Source: CAD feature listing. Evaluate the final solid. Frame: model axes, mm. Round coordinates to 2 decimals unless told otherwise and drop trailing zeros. Loops run counter-clockwise (first coordinate to the right, second up) from the corner with the lowest first, then second, coordinate; pieces in that order, holes last. Notation, with made-up numbers: (4, -15.75) - (35, -15.75) arc R19 cw to (35, 13.25) - close; hole circle Ø9 at (-24, -16.75). An arc over 180 degrees is marked (long way). One line per question, with ' | ' between items.
from build123d import *

# Parameters (mm, degrees)
F4_DEPTH = 3


with BuildPart() as f1:
    # F0 (on Front) → F1 (revolve)
    with BuildSketch(Plane.XZ):
        with BuildLine():
            Line((0, 4), (0, 3))
            Line((0, 3), (6, 3))
            Line((6, 3), (6, 3.356940629))
            ThreePointArc((6, 3.356940629), (5.9878870105, 3.3895684458), (5.9574170226, 3.4063874466))
            Line((5.9574170226, 3.4063874466), (3.3333333333, 3.8))
            Line((3.3333333333, 3.8), (2, 4))
            Line((2, 4), (0, 4))
        make_face()
        Polygon((3.3333333333, 4), (2, 4), (3.3333333333, 3.8), align=None)
    revolve(axis=Axis((0, 0, 3.5), (0, 0, 1)))

    # F2: F1 across face


with BuildPart() as f1_1:
    add(f1.part)
    add(f1.part.mirror(Plane.XY.offset(4)))

    # F3: F1 across face


with BuildPart() as f1_2:
    add(f1_1.part)
    add(f1_1.part.mirror(Plane.XY.offset(5)))

    # F4 (add, through all): a face of the model
    f4_faces = [f1_2.faces().sort_by_distance(p)[0] for p in [
        (0, 0, 3),
    ]]
    extrude(f4_faces, amount=F4_DEPTH)


solid = f1_2.part
1. Section query D-D, the plane y = 5. Give the number of separate pieces and of enclosed holes in the cut face, plus the area to 3 significant figures.
Worked out:
separate pieces: 3 | enclosed holes: 0 | area: 33.1 mm2
2. Section query A-A, the plane y = 0. Return loops of the section in (x, z), plus the area to 3 significant figures.
Worked out:
outline: (-6, 0) - (6, 0) - (6, 3.36) arc R0.05 ccw to (5.96, 3.41) - (3.33, 3.8) - (3.33, 4.2) - (5.96, 4.59) arc R0.05 ccw to (6, 4.64) - (6, 5.36) arc R0.05 ccw to (5.96, 5.41) - (3.33, 5.8) - (3.33, 6.2) - (5.96, 6.59) arc R0.05 ccw to (6, 6.64) - (6, 7) - (-6, 7) - (-6, 6.64) arc R0.05 ccw to (-5.96, 6.59) - (-3.33, 6.2) - (-3.33, 5.8) - (-5.96, 5.41) arc R0.05 ccw to (-6, 5.36) - (-6, 4.64) arc R0.05 ccw to (-5.96, 4.59) - (-3.33, 4.2) - (-3.33, 3.8) - (-5.96, 3.41) arc R0.05 ccw to (-6, 3.36) - close | area: 75.5 mm2
3. Mould query, pull axis Z, two halves, no side actions, for faces 1 (the cylindrical face through (-0.723, -3.254, 4.003)), 2 (the flat face through (0, 0, 0)), 3 (the cylindrical face through (-0.723, -3.254, 6.003)), 4 (the cylindrical face through (-6, 0, 5)). Classes: released by +Z, released by -Z, zero draft, split by the parting line, or undercut.
Worked out:
face 1: undercut | face 2: released by -Z | face 3: undercut | face 4: zero draft
4. Section query C-C, the plane z = 1.75. Return loops of the section in (x, y), plus the area to 3 significant figures.
Worked out:
outline: circle Ø12 at (0, 0) | area: 113 mm2
5. Contact query for flat-ended pins moving along their axis: P1, Ø4, axis at x = -0.5, z = 6, coming from the +Y side; P2, Ø3, axis at x = 3.5, z = 1, coming from the +Y side; P3, Ø1, axis at y = -1.5, z = 2.5, coming from the -X side; P4, Ø2, axis at y = 5, z = 4, coming from the +X side. Output: stop coordinate, or through.
Worked out:
P1: stops at y = 6 | P2: stops at y = 5.66 | P3: stops at x = -5.92 | P4: stops at x = 4.26
6. Material intervals for probe 1 along Z at (x, y) = (5.25, 0.75); probe 2 along Z at (x, y) = (-2.5, 3); probe 3 along Y at (x, z) = (-4.25, 0.5), sorted ascending.
Worked out:
probe 1: z = 0 to 3.5, 4.5 to 5.5, 6.5 to 7 | probe 2: z = 0 to 3.71, 4.29 to 5.71, 6.29 to 7 | probe 3: y = -4.24 to 4.24
